Part model, mm, in its own coordinate system. A direction names the side the tool comes from. Round coordinates to 2 decimals unless told otherwise and drop trailing zeros. Write each loop counter-clockwise with the first axis right and the second up, starting at its lowest first coordinate (ties: lowest second). Pieces come first, ordered by that corner, then holes. Notation, with made-up numbers: (-14.75, 76.5) -> (24.25, 76.5) arc R11 cw to (24.25, 92.5) -> close; hole circle Ø1 at (-31.75, -0.75). An arc over 180 degrees is marked (long way). Use CSV: the item, a comma, the result in double quotes. Start each with the question number.
(1) Two-plate mould, pull along Z, no slides. Class faces 1 (the flat face through (-23, 7, 43.18)), 2 (the flat face through (1, -2.286, -22)), 3 (the flat face through (-29.21, -1, 0)), 4 (the flat face through (1, 0.254, 22)): released by +Z, released by -Z, zero draft, split by the parting line, or undercut.
(2) Saw through at A-A (z = -16.5). Give the cut face in (x, y).
(3) Saw through at D-D (x = 1). Give the cut face in (y, z).
(4) Saw through at C-C (y = 4). Give the cut face in (x, z) (3 decimals).
(5) Saw through at B-B (x = 7.5). Give the cut face in (y, z).
(6) Probe line 1 (Z direction, x = 14, y = -0.5); line 2 (Y direction, x = 2, z = -23); line 3 (Y direction, x = 17.5, z = -33). List the from-to ranges inside material, lowest first. Write a range as [from, to].
(7) Which spindle directions (+Z, -Z, +X, -X, +Y, -Y) get a long thin tool onto all of the face, cutting with end or side? Do faces 5 (the flat face through (19.105, 7, 44)), 6 (the flat face through (29.21, 7, 0)), 7 (the flat face through (26.162, 12, 0)), 8 (the flat face through (1, -1, 15.24)). Say none if no direction does.
(8) Drop flat-ended pins along their axis: pin 1 (1 mm diameter, centred on x = -20, y = 5, fed in from -Z); pin 2 (1 mm diameter, centred on y = 6.5, z = -5, fed in from -X); pin 3 (5.5 mm diameter, centred on y = 7, z = 44, fed in from +X); pin 4 (1.5 mm diameter, centred on y = 9.5, z = 42, fed in from +X). Give the stop position or say it passes through.
```python
from build123d import *

# Parameters (mm, degrees)
SKETCH1_W             = 58.42
SKETCH1_H             = 86.36
BASEPLATE_DEPTH       = 2.032
SKETCH5_W             = 7.62
SKETCH5_H             = 2.032
BOSS_EXTRUDE3_DEPTH   = 9.271
SKETCH5_W_2           = 7.656133635
BOSS_EXTRUDE3_2_DEPTH = 9.271
SKETCH5_W_3           = 7.565007612
BOSS_EXTRUDE3_3_DEPTH = 9.271
SKETCH5_W_4           = 2.032
SKETCH5_H_2           = 12.7
BOSS_EXTRUDE3_4_DEPTH = 9.271
SKETCH5_2_W           = 7.62
SKETCH5_2_H           = 2.032
SKETCH5_2_W_2         = 7.656133635
SKETCH5_2_W_3         = 7.565007612
SKETCH5_2_W_4         = 2.032
SKETCH5_2_H_2         = 12.7
BOSS_EXTRUDE4_DEPTH   = 2.032
SKETCH6_W             = 7.565007612
SKETCH6_H             = 1.778
BOSS_EXTRUDE5_DEPTH   = 3.048
SKETCH6_W_2           = 7.62
BOSS_EXTRUDE5_2_DEPTH = 3.048
BOSS_EXTRUDE5_3_DEPTH = 3.048
SKETCH6_2_W           = 7.565007612
SKETCH6_2_H           = 1.778
SKETCH6_2_W_2         = 7.62
BOSS_EXTRUDE6_DEPTH   = 2.032
SKETCH7_W             = 15.203866365
SKETCH7_H             = 2.032
SKETCH7_W_2           = 15.294992388
SKETCH7_W_3           = 2.54
SKETCH7_W_4           = 2.032
SKETCH7_H_2           = 36.817012066
BOSS_EXTRUDE7_DEPTH   = 2.032
SKETCH9_W             = 12.7
SKETCH9_H             = 1.778
BOSS_EXTRUDE8_DEPTH   = 3.048
SKETCH9_2_W           = 12.7
SKETCH9_2_H           = 1.778
BOSS_EXTRUDE9_DEPTH   = 2.032
SKETCH11_W            = 60.452
SKETCH11_H            = 88.392
BOSS_EXTRUDE10_DEPTH  = 4.064
SKETCH12_W            = 12.7
SKETCH12_H            = 2.54
CUT_EXTRUDE1_DEPTH    = 77.613848676


with BuildPart() as part:
    # Sketch1 → basePlate (new body)
    with BuildSketch(Plane(origin=(0, 0, 0), x_dir=(1, 0, 0), z_dir=(0, 1, 0))):
        Rectangle(SKETCH1_W, SKETCH1_H)
    extrude(amount=BASEPLATE_DEPTH)



with BuildPart() as body_2:
    # Sketch5 → Boss-Extrude3 (new body)
    with BuildSketch(Plane(origin=(0, 2.032, 0), x_dir=(1, 0, 0), z_dir=(0, 1, 0))):
        with Locations((0, -44.196)):
            Rectangle(SKETCH5_W, SKETCH5_H)
    extrude(amount=BOSS_EXTRUDE3_DEPTH)


with BuildPart() as body_3:
    # Sketch5 → Boss-Extrude3 2 (new body)
    with BuildSketch(Plane(origin=(0, 2.032, 0), x_dir=(1, 0, 0), z_dir=(0, 1, 0))):
        with Locations((-22.841933183, -44.196)):
            Rectangle(SKETCH5_W_2, SKETCH5_H)
    extrude(amount=BOSS_EXTRUDE3_2_DEPTH)


with BuildPart() as body_4:
    # Sketch5 → Boss-Extrude3 3 (new body)
    with BuildSketch(Plane(origin=(0, 2.032, 0), x_dir=(1, 0, 0), z_dir=(0, 1, 0))):
        with Locations((22.887496194, -44.196)):
            Rectangle(SKETCH5_W_3, SKETCH5_H)
    extrude(amount=BOSS_EXTRUDE3_3_DEPTH)


with BuildPart() as body_5:
    # Sketch5 → Boss-Extrude3 4 (new body)
    with BuildSketch(Plane(origin=(0, 2.032, 0), x_dir=(1, 0, 0), z_dir=(0, 1, 0))):
        with Locations((30.226, 0.012987934)):
            Rectangle(SKETCH5_W_4, SKETCH5_H_2)
    extrude(amount=BOSS_EXTRUDE3_4_DEPTH)


with BuildPart() as part_1:
    add(part.part)

    add(body_2.part)  # Boss-Extrude4 merges body 2

    add(body_3.part)  # Boss-Extrude4 merges body 3

    add(body_4.part)  # Boss-Extrude4 merges body 4

    add(body_5.part)  # Boss-Extrude4 merges body 5
    # Sketch5<2> → Boss-Extrude4 (add)
    with BuildSketch(Plane(origin=(0, 2.032, 0), x_dir=(1, 0, 0), z_dir=(0, 1, 0))):
        with Locations((0, -44.196)):
            Rectangle(SKETCH5_2_W, SKETCH5_2_H)
        with Locations((-22.841933183, -44.196)):
            Rectangle(SKETCH5_2_W_2, SKETCH5_2_H)
        with Locations((22.887496194, -44.196)):
            Rectangle(SKETCH5_2_W_3, SKETCH5_2_H)
        with Locations((30.226, 0.012987934)):
            Rectangle(SKETCH5_2_W_4, SKETCH5_2_H_2)
    extrude(amount=-BOSS_EXTRUDE4_DEPTH)



with BuildPart() as body_2_2:
    # Sketch6 → Boss-Extrude5 (new body)
    with BuildSketch(Plane(origin=(0, 0, 43.18), x_dir=(-1, 0, 0), z_dir=(0, 0, -1))):
        with Locations((-22.887496194, 12.192)):
            Rectangle(SKETCH6_W, SKETCH6_H)
    extrude(amount=BOSS_EXTRUDE5_DEPTH)


with BuildPart() as body_3_2:
    # Sketch6 → Boss-Extrude5 2 (new body)
    with BuildSketch(Plane(origin=(0, 0, 43.18), x_dir=(-1, 0, 0), z_dir=(0, 0, -1))):
        with Locations((0, 12.192)):
            Rectangle(SKETCH6_W_2, SKETCH6_H)
    extrude(amount=BOSS_EXTRUDE5_2_DEPTH)


with BuildPart() as body_4_2:
    # Sketch6 → Boss-Extrude5 3 (new body)
    with BuildSketch(Plane(origin=(0, 0, 43.18), x_dir=(-1, 0, 0), z_dir=(0, 0, -1))):
        with Locations((22.823866365, 12.192)):
            Rectangle(SKETCH6_W_2, SKETCH6_H)
    extrude(amount=BOSS_EXTRUDE5_3_DEPTH)


with BuildPart() as part_2:
    add(part_1.part)

    add(body_2_2.part)  # Boss-Extrude6 merges body 2 2

    add(body_3_2.part)  # Boss-Extrude6 merges body 3 2

    add(body_4_2.part)  # Boss-Extrude6 merges body 4 2
    # Sketch6<2> → Boss-Extrude6 (add)
    with BuildSketch(Plane(origin=(0, 0, 43.18), x_dir=(-1, 0, 0), z_dir=(0, 0, -1))):
        with Locations((-22.887496194, 12.192)):
            Rectangle(SKETCH6_2_W, SKETCH6_2_H)
        with Locations((0, 12.192)):
            Rectangle(SKETCH6_2_W_2, SKETCH6_2_H)
        with Locations((22.823866365, 12.192)):
            Rectangle(SKETCH6_2_W_2, SKETCH6_2_H)
    extrude(amount=-BOSS_EXTRUDE6_DEPTH)

    # Sketch7 → Boss-Extrude7 (add)
    with BuildSketch(Plane.XZ):
        with Locations((-11.411933183, 44.196)):
            Rectangle(SKETCH7_W, SKETCH7_H)
        with Locations((11.457496194, 44.196)):
            Rectangle(SKETCH7_W_2, SKETCH7_H)
        with Locations((-27.94, 44.196)):
            Rectangle(SKETCH7_W_3, SKETCH7_H)
        Polygon((29.21, 43.18), (26.67, 43.18), (26.67, 45.212), (29.21, 45.212), (31.242, 45.212), (31.242, 6.337012066), (29.21, 6.337012066), align=None)
        with Locations((30.226, -24.771493967)):
            Rectangle(SKETCH7_W_4, SKETCH7_H_2)
    extrude(amount=-BOSS_EXTRUDE7_DEPTH)



with BuildPart() as body_2_3:
    # Sketch9 → Boss-Extrude8 (new body)
    with BuildSketch(Plane.ZY.offset(-29.21)):
        with Locations((-0.012987934, 12.192)):
            Rectangle(SKETCH9_W, SKETCH9_H)
    extrude(amount=BOSS_EXTRUDE8_DEPTH)


with BuildPart() as part_3:
    add(part_2.part)

    add(body_2_3.part)  # Boss-Extrude9 merges body 2 3
    # Sketch9<2> → Boss-Extrude9 (add)
    with BuildSketch(Plane.ZY.offset(-29.21)):
        with Locations((-0.012987934, 12.192)):
            Rectangle(SKETCH9_2_W, SKETCH9_2_H)
    extrude(amount=-BOSS_EXTRUDE9_DEPTH)

    # Sketch11 → Boss-Extrude10 (add)
    with BuildSketch(Plane.XZ):
        with Locations((1.016, 1.016)):
            Rectangle(SKETCH11_W, SKETCH11_H)
    extrude(amount=BOSS_EXTRUDE10_DEPTH)

    # Sketch12 → Cut-Extrude1 (cut, through all)
    with BuildSketch(Plane.ZY.offset(29.21)):
        with Locations((-21.59, -1.016)):
            Rectangle(SKETCH12_W, SKETCH12_H)
        with Locations((21.59, -1.016)):
            Rectangle(SKETCH12_W, SKETCH12_H)
    extrude(amount=-CUT_EXTRUDE1_DEPTH, mode=Mode.SUBTRACT)


solid = part_3.part
```
Answers:
1,face 1,"released by -Z"
1,face 2,"undercut"
1,face 3,"zero draft"
1,face 4,"undercut"
2,outline,"(-29.21, -4.06) -> (31.24, -4.06) -> (31.24, -2.29) -> (-29.21, -2.29) -> close; (-29.21, 0.25) -> (31.24, 0.25) -> (31.24, 2.03) -> (-29.21, 2.03) -> close"
3,outline,"(-4.06, -43.18) -> (2.03, -43.18) -> (2.03, 43.18) -> (11.3, 43.18) -> (11.3, 40.13) -> (13.08, 40.13) -> (13.08, 45.21) -> (-4.06, 45.21) -> close; hole (-2.29, -27.94) -> (0.25, -27.94) -> (0.25, -15.24) -> (-2.29, -15.24) -> close; hole (-2.29, 15.24) -> (0.25, 15.24) -> (0.25, 27.94) -> (-2.29, 27.94) -> close"
4,outline,"(-26.67, 43.18) -> (-19.014, 43.18) -> (-19.014, 45.212) -> (-26.67, 45.212) -> close; (-3.81, 43.18) -> (3.81, 43.18) -> (3.81, 45.212) -> (-3.81, 45.212) -> close; (19.105, 43.18) -> (26.67, 43.18) -> (26.67, 45.212) -> (19.105, 45.212) -> close; (29.21, -6.363) -> (31.242, -6.363) -> (31.242, 6.337) -> (29.21, 6.337) -> close"
5,outline,"(-4.06, -43.18) -> (2.03, -43.18) -> (2.03, 45.21) -> (-4.06, 45.21) -> close; hole (-2.29, -27.94) -> (0.25, -27.94) -> (0.25, -15.24) -> (-2.29, -15.24) -> close; hole (-2.29, 15.24) -> (0.25, 15.24) -> (0.25, 27.94) -> (-2.29, 27.94) -> close"
6,line 1,"z = [-43.18, -27.94], [-15.24, 15.24], [27.94, 45.21]"
6,line 2,"y = [-4.06, -2.29], [0.25, 2.03]"
6,line 3,"y = [-4.06, 2.03]"
7,face 5,"+Z, -Z, +Y"
7,face 6,"+Z, -Z, -X"
7,face 7,"-Z, -X, +Y"
7,face 8,"+X, -X"
8,pin 1,"stops at z = 43.18"
8,pin 2,"stops at x = 29.21"
8,pin 3,"stops at x = 26.67"
8,pin 4,"passes through"
